Geometry: final body of the model. Coordinates: model frame, mm. Coordinates: 2 decimals unless noted, no trailing zeros. Write each loop counter-clockwise with the first axis right and the second up, starting at its lowest first coordinate (ties: lowest second). Pieces come first, ordered by that corner, then holes.
from build123d import *

# Parameters (mm, degrees)
SKETCH1_W           = 603.25
SKETCH1_H           = 88.9
BOSS_EXTRUDE1_DEPTH = 2.54
SKETCH2_W           = 25.4
SKETCH2_H           = 25.4
CUT_EXTRUDE1_DEPTH  = 5.08
SKETCH3_R           = 1.63195
CUT_EXTRUDE2_DEPTH  = 5.08
SKETCH4_R           = 1.63195
CUT_EXTRUDE3_DEPTH  = 5.08
LPATTERN1_COUNT     = 2
LPATTERN1_PITCH     = 70.104


with BuildPart() as part:
    # Sketch1 → Boss-Extrude1 (new body, symmetric)
    with BuildSketch(Plane.XY):
        Rectangle(SKETCH1_W, SKETCH1_H)
    extrude(amount=BOSS_EXTRUDE1_DEPTH, both=True)

    # Sketch2 → Cut-Extrude1 (cut)
    with BuildSketch(Plane.XY.offset(2.54)):
        with Locations((-288.925, 31.75)):
            Rectangle(SKETCH2_W, SKETCH2_H)
        with Locations((288.925, 31.75)):
            Rectangle(SKETCH2_W, SKETCH2_H)
        with Locations((12.7, 31.75)):
            Rectangle(SKETCH2_W, SKETCH2_H)
        with Locations((12.7, -31.75)):
            Rectangle(SKETCH2_W, SKETCH2_H)
    extrude(amount=-CUT_EXTRUDE1_DEPTH, mode=Mode.SUBTRACT)

    # Sketch3 → Cut-Extrude2 (cut)
    with BuildSketch(Plane.XY.offset(2.54)):
        with Locations((-14.478, 30.099)):
            Circle(SKETCH3_R)
        with Locations((-30.226, 33.401)):
            Circle(SKETCH3_R)
    cut_extrude2 = extrude(amount=-CUT_EXTRUDE2_DEPTH, mode=Mode.SUBTRACT)

    # Sketch4 → Cut-Extrude3 (cut)
    with BuildSketch(Plane.XY.offset(2.54)):
        with Locations((-290.576, 4.572)):
            Circle(SKETCH4_R)
        with Locations((-287.274, -11.176)):
            Circle(SKETCH4_R)
    cut_extrude3 = extrude(amount=-CUT_EXTRUDE3_DEPTH, mode=Mode.SUBTRACT)

    # Mirror2: Cut-Extrude3 across plane
    add(cut_extrude3.mirror(Plane(origin=(0, 0, 0), x_dir=(0, 0, 1), z_dir=(1, 0, 0))), mode=Mode.SUBTRACT)

    # LPattern1: Cut-Extrude2 ×2
    with Locations(*[(i * LPATTERN1_PITCH, 0, 0) for i in range(1, LPATTERN1_COUNT)]):
        add(cut_extrude2, mode=Mode.SUBTRACT)


solid = part.part
Item 1: Section B-B, the plane z = -0.8. State how many separate pieces and enclosed holes the cut face has, plus the area to 3 significant figures.
Derived:
separate pieces: 1
enclosed holes: 8
area: 51,000 mm2
Item 2: Pin query (flat end, axial travel): pin 1 (1.5 mm diameter, centred on y = 20.5, z = 0.5, fed in from -X) (3 decimals); pin 2 (1.5 mm diameter, centred on y = 34.5, z = 1, fed in from +X) (3 decimals). Return the tip coordinate at first contact, or that it passes through.
Derived:
pin 1: stops at x = -276.225
pin 2: stops at x = 276.225
Item 3: Material intervals for probe 1 along X at (y, z) = (30, -0.4) (3 decimals); probe 2 along X at (y, z) = (39.5, 0.3) (3 decimals); probe 3 along X at (y, z) = (-26.5, 0.3) (3 decimals), sorted ascending.
Derived:
probe 1: x = -276.225 to -16.107, -12.849 to 0, 25.4 to 53.997, 57.255 to 276.225
probe 2: x = -276.225 to 0, 25.4 to 276.225
probe 3: x = -301.625 to 0, 25.4 to 301.625
Item 4: Section A-A, the plane y = -36.5. Output: boundary loops of the cut face in (x, z) (3 decimals).
Derived:
outline: (-301.625, -2.54) - (0, -2.54) - (0, 2.54) - (-301.625, 2.54) - close; (25.4, -2.54) - (301.625, -2.54) - (301.625, 2.54) - (25.4, 2.54) - close
Item 5: Section C-C, the plane x = 6. Output: boundary loops of the cut face in (y, z), plus the area to 3 significant figures.
Derived:
outline: (-19.05, -2.54) - (19.05, -2.54) - (19.05, 2.54) - (-19.05, 2.54) - close
area: 194 mm2
Item 6: Pull-direction query (Z, two-part tool) for faces 1 (the flat face through (-4, 1, -2.54)), 2 (the flat face through (-4, 1, 2.54)); classes: released by +Z, released by -Z, zero draft, split by the parting line, or undercut.
Derived:
face 1: released by -Z
face 2: released by +Z
